from build123d import *

# Parameters (mm, degrees)
BOSS_EXTRUDE1_DEPTH = 95.25
SKETCH3_R           = 3.175
CUT_EXTRUDE1_DEPTH  = 26.366155757
SKETCH4_R           = 4
SKETCH4_R_2         = 1.75
CUT_EXTRUDE2_DEPTH  = 26.366155757
LPATTERN1_COUNT     = 2
LPATTERN1_PITCH     = 16
LPATTERN1_COL_COUNT = 2
LPATTERN1_COL_PITCH = 16
SKETCH5_W           = 44.45
SKETCH5_H           = 63.5
CUT_EXTRUDE3_DEPTH  = 26.366155757
SKETCH6_W           = 25.4
SKETCH6_H           = 63.5
CUT_EXTRUDE4_DEPTH  = 26.366155757
SKETCH8_W           = 6.35
SKETCH8_H           = 12.7
CUT_EXTRUDE6_DEPTH  = 26.366155757
LPATTERN2_COUNT     = 18
LPATTERN2_PITCH     = 25.4
SKETCH9_W           = 12.7
SKETCH9_H           = 6.403441613
CUT_EXTRUDE7_DEPTH  = 26.366155757
SKETCH10_W          = 12.7
SKETCH10_H          = 6.35
CUT_EXTRUDE8_DEPTH  = 26.366155757


with BuildPart() as part:
    # Sketch2 → Boss-Extrude1 (new body)
    with BuildSketch(Plane.XY):
        Polygon((38.583668647, 0.58465909), (44.904434507, -0.023961438), (64.008541785, 198.379778502), (57.687775925, 198.988399031), align=None)
    extrude(amount=BOSS_EXTRUDE1_DEPTH)

    # Sketch3 → Cut-Extrude1 (cut, through all)
    with BuildSketch(Plane(origin=(38.173444207, -3.675684609, 0), x_dir=(0, 0, 1), z_dir=(-0.995396198, 0.095845753, 0))):
        with Locations((9.525, 20.155048192)):
            Circle(SKETCH3_R)
        with Locations((85.725, 20.155048192)):
            Circle(SKETCH3_R)
    extrude(amount=-CUT_EXTRUDE1_DEPTH, mode=Mode.SUBTRACT)

    # Sketch4 → Cut-Extrude2 (cut, through all)
    with BuildSketch(Plane(origin=(38.173444207, -3.675684609, 0), x_dir=(0, 0, 1), z_dir=(-0.995396198, 0.095845753, 0))):
        with Locations((47.625, 105.880048192)):
            Circle(SKETCH4_R)
        with Locations((47.625, 113.880048192)):
            Circle(SKETCH4_R_2)
        with Locations((55.625, 105.880048192)):
            Circle(SKETCH4_R_2)
        with Locations((47.625, 97.880048192)):
            Circle(SKETCH4_R_2)
        with Locations((39.625, 105.880048192)):
            Circle(SKETCH4_R_2)
    cut_extrude2 = extrude(amount=-CUT_EXTRUDE2_DEPTH, mode=Mode.SUBTRACT)

    # LPattern1: Cut-Extrude2 ×2
    with Locations(*[(0, 0, i * LPATTERN1_PITCH) for i in range(1, LPATTERN1_COUNT)]):
        add(cut_extrude2, mode=Mode.SUBTRACT)

    # LPattern1 col: Cut-Extrude2 ×2
    with Locations(*[(0, 0, -i * LPATTERN1_COL_PITCH) for i in range(1, LPATTERN1_COL_COUNT)]):
        add(cut_extrude2, mode=Mode.SUBTRACT)

    # Sketch5 → Cut-Extrude3 (cut, through all)
    with BuildSketch(Plane(origin=(38.173444207, -3.675684609, 0), x_dir=(0, 0, 1), z_dir=(-0.995396198, 0.095845753, 0))):
        with Locations((47.625, 153.630048192)):
            Rectangle(SKETCH5_W, SKETCH5_H)
    extrude(amount=-CUT_EXTRUDE3_DEPTH, mode=Mode.SUBTRACT)

    # Sketch6 → Cut-Extrude4 (cut, through all)
    with BuildSketch(Plane(origin=(38.173444207, -3.675684609, 0), x_dir=(0, 0, 1), z_dir=(-0.995396198, 0.095845753, 0))):
        with Locations((31.75, 36.030048192)):
            Rectangle(SKETCH6_W, SKETCH6_H)
    extrude(amount=-CUT_EXTRUDE4_DEPTH, mode=Mode.SUBTRACT)

    # Sketch8 → Cut-Extrude6 (cut, through all)
    with BuildSketch(Plane(origin=(38.173444207, -3.675684609, 0), x_dir=(0, 0, 1), z_dir=(-0.995396198, 0.095845753, 0))):
        with Locations((3.175, 10.630048192)):
            Rectangle(SKETCH8_W, SKETCH8_H)
        with Locations((92.075, 10.630048192)):
            Rectangle(SKETCH8_W, SKETCH8_H)
    cut_extrude6 = extrude(amount=-CUT_EXTRUDE6_DEPTH, mode=Mode.SUBTRACT)

    # LPattern2: Cut-Extrude6 ×18
    with Locations(*[Vector(0.095845753, 0.995396198, 0) * (i * LPATTERN2_PITCH) for i in range(1, LPATTERN2_COUNT)]):
        add(cut_extrude6, mode=Mode.SUBTRACT)

    # Sketch9 → Cut-Extrude7 (cut, through all)
    with BuildSketch(Plane(origin=(38.173444207, -3.675684609, 0), x_dir=(0, 0, 1), z_dir=(-0.995396198, 0.095845753, 0))):
        with Locations((63.5, 7.481768999)):
            Rectangle(SKETCH9_W, SKETCH9_H)
    extrude(amount=-CUT_EXTRUDE7_DEPTH, mode=Mode.SUBTRACT)

    # Sketch10 → Cut-Extrude8 (cut, through all)
    with BuildSketch(Plane(origin=(38.173444207, -3.675684609, 0), x_dir=(0, 0, 1), z_dir=(-0.995396198, 0.095845753, 0))):
        with Locations((19.05, 200.426424209)):
            Rectangle(SKETCH10_W, SKETCH10_H)
        with Locations((47.625, 200.426424209)):
            Rectangle(SKETCH10_W, SKETCH10_H)
        with Locations((76.2, 200.426424209)):
            Rectangle(SKETCH10_W, SKETCH10_H)
    extrude(amount=-CUT_EXTRUDE8_DEPTH, mode=Mode.SUBTRACT)


solid = part.part
Model file for the job. Use its own axes, mm. A direction names the side the tool comes from. Round coordinates to 2 decimals unless told otherwise and drop trailing zeros. Loops run counter-clockwise (first coordinate to the right, second up) from the corner with the lowest first, then second, coordinate; pieces in that order, holes last.
1. Drop flat-ended pins along their axis: P1, Ø8.5, axis at x = 44, y = 31, coming from the +Z side; P2, Ø1, axis at x = 55, z = 37.5, coming from the +Y side; P3, Ø7.5, axis at x = 60, y = 194.5, coming from the -Z side; P4, Ø6, axis at x = 43, y = 30.5, coming from the -Z side. Give the stop position or say it passes through.
Check values:
P1: stops at z = 88.9
P2: stops at y = 117.2
P3: stops at z = 0
P4: stops at z = 6.35
2. Mould opens along Y. For faces 4 (the flat face through (60.195, 192.368, 18.961)), 5 (the flat face through (59, 183, 6.35)), 6 (the cylindrical face through (50.607, 92.787, 65.242)), 7 (the flat face through (60, 194, 0)) say: +Y half, -Y half, draft (parallel to the pull), parting line (faces both ways), or undercut.
Check values:
face 4: +Y half
face 5: undercut
face 6: undercut
face 7: draft
3. Band-saw the part on A-A, the plane y = 45. List the corners of the cut face in (x, z).
Check values:
outline: (42.86, 0) - (49.24, 0) - (49.24, 19.05) - (42.86, 19.05) - close; (42.86, 44.45) - (49.24, 44.45) - (49.24, 95.25) - (42.86, 95.25) - close
4. Band-saw the part on B-B, the plane z = 80. List the corners of the cut face in (x, y), and give its area (3 significant figures).
Check values:
outline: (38.58, 0.58) - (44.9, -0.02) - (63.4, 192.06) - (57.08, 192.67) - close
area: 1,230 mm2
5. Tool access for faces 1 (the flat face through (56.307, 151.983, 92.031)), 2 (the flat face through (45.35, 38.21, 3.13)), 3 (the flat face through (45, 31, 44.45)): list every direction of +Z, -Z, +X, -X, +Y, -Y with a clear straight run to the whole face (end or side of a thin tool).
Check values:
face 1: +Z, +X
face 2: -Z, -X
face 3: +X, -X, -Y
6. Wall check: probe 1 along Z at (x, y) = (47.25, 62); probe 2 along Y at (x, z) = (50.25, 28); probe 3 along X at (y, z) = (190, 36). Give the ranges that are in metal, low to high.
Check values:
probe 1: z = 6.35 to 19.05, 44.45 to 88.9
probe 2: y = 63.26 to 99.83, 103.23 to 117.61
probe 3: x = 56.82 to 63.2
